from build123d import *

# Parameters (mm, degrees)
F0_W      = 476.25
F0_H      = 152.4
F1_DEPTH  = 38.1
F2_W      = 209.55
F2_H      = 152.4
F3_DEPTH  = 12.7
F5_DEPTH  = 38.101
F7_D      = 7.9375
F8_D      = 5.1054
F9_W      = 19.05
F9_H      = 88.9
F10_DEPTH = 38.1
F12_D     = 13.49248


with BuildPart() as f1:
    # F0 (on Top) → F1 (new body)
    with BuildSketch(Plane.XY):
        Rectangle(F0_W, F0_H)
    extrude(amount=F1_DEPTH)

    # F2 (on face) → F3 (cut)
    with BuildSketch(Plane.XY.offset(38.1)):
        with Locations((133.35, 0)):
            Rectangle(F2_W, F2_H)
    extrude(amount=-F3_DEPTH, mode=Mode.SUBTRACT)

    # F4 (on face) → F5 (cut, through all)
    with BuildSketch(Plane.XY.offset(38.1)):
        with BuildLine():
            Line((3.175, -43.65625), (-34.925, -43.65625))
            ThreePointArc((-34.925, -43.65625), (-42.06875, -50.8), (-34.925, -57.94375))
            Line((-34.925, -57.94375), (3.175, -57.94375))
            ThreePointArc((3.175, -57.94375), (10.31875, -50.8), (3.175, -43.65625))
        make_face()
        with BuildLine():
            Line((219.075, -43.65625), (180.975, -43.65625))
            ThreePointArc((180.975, -43.65625), (173.83125, -50.8), (180.975, -57.94375))
            Line((180.975, -57.94375), (219.075, -57.94375))
            ThreePointArc((219.075, -57.94375), (226.21875, -50.8), (219.075, -43.65625))
        make_face()
        with BuildLine():
            ThreePointArc((-34.925, 57.94375), (-42.06875, 50.8), (-34.925, 43.65625))
            Line((-34.925, 43.65625), (3.175, 43.65625))
            ThreePointArc((3.175, 43.65625), (10.31875, 50.8), (3.175, 57.94375))
            Line((3.175, 57.94375), (-34.925, 57.94375))
        make_face()
        with BuildLine():
            ThreePointArc((180.975, 57.94375), (173.83125, 50.8), (180.975, 43.65625))
            Line((180.975, 43.65625), (219.075, 43.65625))
            ThreePointArc((219.075, 43.65625), (226.21875, 50.8), (219.075, 57.94375))
            Line((219.075, 57.94375), (180.975, 57.94375))
        make_face()
    extrude(amount=-F5_DEPTH, mode=Mode.SUBTRACT)

    # F7 (through all)
    with Locations(Plane.XY.offset(38.1)):
        with Locations((-174.625, 51.562), (-71.501, 51.562), (-174.625, -51.562), (-71.501, -51.562)):
            Hole(F7_D / 2)

    # F8 (through all)
    with Locations(Plane.XY.offset(38.1)):
        with Locations((88.011, 53.848), (157.861, 53.848), (88.011, -53.848), (157.861, -53.848)):
            Hole(F8_D / 2)

    # F9 (on face) → F10 (join)
    with BuildSketch(Plane(origin=(0, 0, 0), x_dir=(1, 0, 0), z_dir=(0, 0, -1))):
        with Locations((-215.9, 0)):
            Rectangle(F9_W, F9_H)
    extrude(amount=F10_DEPTH)

    # F12 (through all)
    with Locations(Plane(origin=(-225.425, 0, 0), x_dir=(0, -1, 0), z_dir=(-1, 0, 0))):
        with Locations((-31.75, -25.4), (31.75, -25.4)):
            Hole(F12_D / 2)


solid = f1.part
Source: CAD feature listing. Evaluate the final solid. Frame: model axes, mm. A direction names the side the tool comes from. Coordinates: 2 decimals unless noted, no trailing zeros. Loops run counter-clockwise (first coordinate to the right, second up) from the corner with the lowest first, then second, coordinate; pieces in that order, holes last. Notation, with made-up numbers: M 12,-9.5 L 62,-9.5 A25 ccw 62,10.5 Z; hole C 68.5,48.5 d9. An arc over 180 degrees is marked long. Answer in a Markdown table with one row per item.
Q1. Section A-A on z = -25.4. Return the cut outline in (x, y) (3 decimals).
Answers below:
| item | result |
|---|---|
| outline | M -225.425,-44.45 L -206.375,-44.45 L -206.375,-38.496 L -225.425,-38.496 Z; M -225.425,-25.004 L -206.375,-25.004 L -206.375,25.004 L -225.425,25.004 Z; M -225.425,38.496 L -206.375,38.496 L -206.375,44.45 L -225.425,44.45 Z |
Q2. Draft query along Y for faces 1 (the flat face through (238.125, -1, 13)), 2 (the cylindrical face through (173.833, -50.643, 12.878)), 3 (the flat face through (-3, -76.2, 15)). Return one class per face: pulls with the +Y half, pulls with the -Y half, needs draft (parallel to the pull), parting line crosses it, or undercut.
Answers below:
| item | result |
|---|---|
| face 1 | needs draft |
| face 2 | undercut |
| face 3 | pulls with the -Y half |
Q3. Set-up query: faces 4 (the flat face through (132, 1, 25.4)), 5 (the cylindrical face through (10.317, -50.957, 19.317)), 6 (the flat face through (-238.125, -1, 19)). Return all of +Z, -Z, +X, -X, +Y, -Y with unobstructed straight access to the full face (end or side cutting, diameter ignored); none if empty.
Answers below:
| item | result |
|---|---|
| face 4 | +Z, +X, +Y, -Y |
| face 5 | +Z, -Z |
| face 6 | +Z, -Z, -X, +Y, -Y |
Q4. Section D-D on x = 22. Return the cut outline in (y, z), plus the area to 3 significant figures.
Answers below:
| item | result |
|---|---|
| outline | M -76.2,0 L 76.2,0 L 76.2,38.1 L -76.2,38.1 Z |
| area | 5,810 mm^2 |
Q5. Section C-C on y = -11.5. Return the cut outline in (x, z) (3 decimals).
Answers below:
| item | result |
|---|---|
| outline | M -238.125,0 L -225.425,0 L -225.425,-38.1 L -206.375,-38.1 L -206.375,0 L 238.125,0 L 238.125,25.4 L 28.575,25.4 L 28.575,38.1 L -238.125,38.1 Z |
Q6. Ray query, probe 1 along Z at (x, y) = (-214.25, -31.75); probe 2 along Z at (x, y) = (-140, 3.5); probe 3 along Z at (x, y) = (140.5, -4.5). Return the intervals inside material, ascending. Write a range as from..to.
Answers below:
| item | result |
|---|---|
| probe 1 | z = -38.1..-32.15, -18.65..38.1 |
| probe 2 | z = 0..38.1 |
| probe 3 | z = 0..25.4 |
Q7. First-contact query: pin 1 (6.5 mm diameter, centred on y = -37.5, z = 29, fed in from +X) (3 decimals); pin 2 (11.5 mm diameter, centred on y = -14.5, z = -13, fed in from -X) (3 decimals); pin 3 (1 mm diameter, centred on x = 77.5, y = -40, fed in from -Z). Flat tips, straight axial feed; report the tip coordinate or a pass-through.
Answers below:
| item | result |
|---|---|
| pin 1 | stops at x = 28.575 |
| pin 2 | stops at x = -225.425 |
| pin 3 | stops at z = 0 |
Q8. Section B-B on y = 31.75. Return the cut outline in (x, z) (3 decimals).
Answers below:
| item | result |
|---|---|
| outline | M -238.125,0 L -225.425,0 L -225.425,-18.654 L -206.375,-18.654 L -206.375,0 L 238.125,0 L 238.125,25.4 L 28.575,25.4 L 28.575,38.1 L -238.125,38.1 Z; M -225.425,-38.1 L -206.375,-38.1 L -206.375,-32.146 L -225.425,-32.146 Z |
